from build123d import *

# Parameters (mm, degrees)
SKETCH2_W             = 152.4
SKETCH2_H             = 50.8
SKETCH2_W_2           = 146.05
SKETCH2_H_2           = 44.45
BOSS_EXTRUDE1_DEPTH   = 1133.475
BOSS_EXTRUDE1_2_DEPTH = 1133.475
BOSS_EXTRUDE4_DEPTH   = 858.8375
SKETCH5_W             = 50.8
SKETCH5_H             = 6.35
BOSS_EXTRUDE5_DEPTH   = 1163.6375
BOSS_EXTRUDE6_DEPTH   = 858.8375
SKETCH7_W             = 101.6
SKETCH7_H             = 101.6
BOSS_EXTRUDE7_DEPTH   = 25.4
SKETCH1_W             = 1143
SKETCH1_H             = 19.05
BOSS_EXTRUDE8_DEPTH   = 12.7
BOSS_EXTRUDE9_DEPTH   = 3.175
SKETCH8_R             = 6.35
CUT_EXTRUDE1_DEPTH    = 2252.98


with BuildPart() as part:
    # Sketch2 → Boss-Extrude1 (new body, symmetric)
    with BuildSketch(Plane(origin=(0, 0, 0), x_dir=(1, 0, 0), z_dir=(0, 1, 0))):
        with Locations((-505.61875, 0)):
            Rectangle(SKETCH2_W, SKETCH2_H)
        with Locations((-505.61875, 0)):
            Rectangle(SKETCH2_W_2, SKETCH2_H_2, mode=Mode.SUBTRACT)
    extrude(amount=BOSS_EXTRUDE1_DEPTH, both=True)



with BuildPart() as body_2:
    # Sketch2 → Boss-Extrude1 2 (new body, symmetric)
    with BuildSketch(Plane(origin=(0, 0, 0), x_dir=(1, 0, 0), z_dir=(0, 1, 0))):
        with Locations((505.61875, 0)):
            Rectangle(SKETCH2_W, SKETCH2_H)
        with Locations((505.61875, 0)):
            Rectangle(SKETCH2_W_2, SKETCH2_H_2, mode=Mode.SUBTRACT)
    extrude(amount=BOSS_EXTRUDE1_2_DEPTH, both=True)


with BuildPart() as part_1:
    add(part.part)

    add(body_2.part)  # Boss-Extrude4 merges body 2
    # Sketch3 → Boss-Extrude4 (add)
    with BuildSketch(Plane.ZY.offset(-429.41875)):
        Polygon((19.05, 987.425), (0, 987.425), (0, 981.075), (25.4, 981.075), (25.4, 1133.475), (-25.4, 1133.475), (-25.4, 1127.125), (19.05, 1127.125), align=None)
        Polygon((-25.4, -1133.475), (25.4, -1133.475), (25.4, -981.075), (0, -981.075), (0, -987.425), (19.05, -987.425), (19.05, -1127.125), (-25.4, -1127.125), align=None)
    extrude(amount=BOSS_EXTRUDE4_DEPTH)

    # Sketch5 → Boss-Extrude5 (add)
    with BuildSketch(Plane.ZY.offset(581.81875)):
        with Locations((0, -1133.475)):
            Rectangle(SKETCH5_W, SKETCH5_H)
        with Locations((0, 1133.475)):
            Rectangle(SKETCH5_W, SKETCH5_H)
    extrude(amount=-BOSS_EXTRUDE5_DEPTH)

    # Sketch6 → Boss-Extrude6 (add)
    with BuildSketch(Plane(origin=(-429.41875, 0, 0), x_dir=(0, 0, -1), z_dir=(1, 0, 0))):
        Polygon((-15.875, -981.075), (-15.875, -482.6), (6.35, -457.2), (6.35, -304.8), (-15.875, -279.4), (-15.875, 279.4), (6.35, 304.8), (6.35, 457.2), (-15.875, 482.6), (-15.875, 981.075), (-22.225, 981.075), (-22.225, 482.6), (0, 457.2), (0, 304.8), (-22.225, 279.4), (-22.225, -279.4), (0, -304.8), (0, -457.2), (-22.225, -482.6), (-22.225, -981.075), align=None)
    extrude(amount=BOSS_EXTRUDE6_DEPTH)

    # Sketch7 → Boss-Extrude7 (add)
    with BuildSketch(Plane.XY.offset(25.4)):
        with Locations((584.2, 1075.69)):
            Rectangle(SKETCH7_W, SKETCH7_H)
        with Locations((584.2, 364.49)):
            Rectangle(SKETCH7_W, SKETCH7_H)
        with Locations((584.2, -364.49)):
            Rectangle(SKETCH7_W, SKETCH7_H)
        with Locations((584.2, -1075.69)):
            Rectangle(SKETCH7_W, SKETCH7_H)
    extrude(amount=-BOSS_EXTRUDE7_DEPTH)

    # Sketch1 → Boss-Extrude8 (add)
    with BuildSketch(Plane.XY):
        with Locations((0, -1133.475)):
            Rectangle(SKETCH1_W, SKETCH1_H)
        with Locations((0, 1133.475)):
            Rectangle(SKETCH1_W, SKETCH1_H)
    extrude(amount=-BOSS_EXTRUDE8_DEPTH)

    # Sketch9 → Boss-Extrude9 (add)
    with BuildSketch(Plane.XY.offset(25.4)):
        with BuildLine():
            Line((635, 1126.49), (635, 1024.89))
            Line((635, 1024.89), (579.538518777, 1024.89))
            ThreePointArc((579.538518777, 1024.89), (572.213815984, 1026.468854084), (566.189972237, 1030.925013611))
            Line((566.189972237, 1030.925013611), (534.1840739, 1067.300724008))
            ThreePointArc((534.1840739, 1067.300724008), (531.01875, 1075.69), (534.1840739, 1084.079275992))
            Line((534.1840739, 1084.079275992), (566.189972237, 1120.454986389))
            ThreePointArc((566.189972237, 1120.454986389), (572.213815984, 1124.911145916), (579.538518777, 1126.49))
            Line((579.538518777, 1126.49), (635, 1126.49))
        make_face()
        with BuildLine():
            Line((635, 415.29), (635, 313.69))
            Line((635, 313.69), (578.904878784, 313.69))
            ThreePointArc((578.904878784, 313.69), (571.5, 315.30534194), (565.440611797, 319.857854871))
            Line((565.440611797, 319.857854871), (534.101416438, 356.195610622))
            ThreePointArc((534.101416438, 356.195610622), (531.01875, 364.49), (534.101416438, 372.784389378))
            Line((534.101416438, 372.784389378), (565.440611797, 409.122145129))
            ThreePointArc((565.440611797, 409.122145129), (571.5, 413.67465806), (578.904878784, 415.29))
            Line((578.904878784, 415.29), (635, 415.29))
        make_face()
        with BuildLine():
            Line((635, -313.69), (635, -415.29))
            Line((635, -415.29), (578.904878784, -415.29))
            ThreePointArc((578.904878784, -415.29), (571.5, -413.67465806), (565.440611797, -409.122145129))
            Line((565.440611797, -409.122145129), (534.101416438, -372.784389378))
            ThreePointArc((534.101416438, -372.784389378), (531.01875, -364.49), (534.101416438, -356.195610622))
            Line((534.101416438, -356.195610622), (565.440611797, -319.857854871))
            ThreePointArc((565.440611797, -319.857854871), (571.5, -315.30534194), (578.904878784, -313.69))
            Line((578.904878784, -313.69), (635, -313.69))
        make_face()
        with BuildLine():
            Line((635, -1024.89), (635, -1126.49))
            Line((635, -1126.49), (578.904878784, -1126.49))
            ThreePointArc((578.904878784, -1126.49), (571.5, -1124.87465806), (565.440611797, -1120.322145129))
            Line((565.440611797, -1120.322145129), (534.101416438, -1083.984389378))
            ThreePointArc((534.101416438, -1083.984389378), (531.01875, -1075.69), (534.101416438, -1067.395610622))
            Line((534.101416438, -1067.395610622), (565.440611797, -1031.057854871))
            ThreePointArc((565.440611797, -1031.057854871), (571.5, -1026.50534194), (578.904878784, -1024.89))
            Line((578.904878784, -1024.89), (635, -1024.89))
        make_face()
    extrude(amount=BOSS_EXTRUDE9_DEPTH)

    # Sketch8 → Cut-Extrude1 (cut)
    with BuildSketch(Plane(origin=(0, 1126.49, 0), x_dir=(1, 0, 0), z_dir=(0, 1, 0))):
        with Locations((619.91875, -12.7)):
            Circle(SKETCH8_R)
        with BuildLine():
            Line((619.91875, 0), (635, 0))
            Line((635, 0), (635, -28.575))
            Line((635, -28.575), (619.91875, -28.575))
            Line((619.91875, -28.575), (619.91875, -25.4))
            ThreePointArc((619.91875, -25.4), (632.61875, -12.7), (619.91875, 0))
        make_face()
    extrude(amount=-CUT_EXTRUDE1_DEPTH, mode=Mode.SUBTRACT)


solid = part_1.part
Work out the finished part from the listing and answer in its coordinate system (mm). A direction names the side the tool comes from. Give positions to 0.01 mm unless a question says otherwise; leave off trailing zeros. Write each loop counter-clockwise with the first axis right and the second up, starting at its lowest first coordinate (ties: lowest second). Pieces come first, ordered by that corner, then holes. Notation, with made-up numbers: M 48.5,27 L 96.5,27 A23 cw 96.5,56 Z; hole C -28.5,66.25 d10. An arc over 180 degrees is marked long. Answer as CSV lines item,"result".
Q1. A cutting plane is placed at A-A on y = -689.5. Write down the section's boundary in (x, z) (3 decimals).
A:
outline,"M -581.819,-25.4 L -429.419,-25.4 L -429.419,15.875 L 429.419,15.875 L 429.419,-25.4 L 581.819,-25.4 L 581.819,25.4 L 429.419,25.4 L 429.419,22.225 L -429.419,22.225 L -429.419,25.4 L -581.819,25.4 Z; hole M -578.644,-22.225 L -432.594,-22.225 L -432.594,22.225 L -578.644,22.225 Z; hole M 432.594,-22.225 L 578.644,-22.225 L 578.644,22.225 L 432.594,22.225 Z"
Q2. A tool of negligible diameter and unlimited length cuts with its end or side. For faces 5 (the flat face through (-6, -382, -6.35)), 6 (the flat face through (432.594, 16, 0)), 7 (the flat face through (586, 365, 28.575)), 8 (the flat face through (-6, -380, 0)), from which of +Z, -Z, +X, -X, +Y, -Y can it reach the whole face along a straight path? Write none if from no direction.
A:
face 5,"-Z"
face 6,"none"
face 7,"+Z, +X, -X, +Y, -Y"
face 8,"+Z"
Q3. The mould has two halves that part along Z. Classify faces 1 (the flat face through (581.819, 16, 0)), 2 (the flat face through (-6, -728, 22.225)), 3 (the flat face through (505, 1130.3, 5)), 4 (the flat face through (505, 16, 22.225)): +Z half, -Z half, draft (parallel to the pull), parting line (faces both ways), or undercut.
A:
face 1,"draft"
face 2,"+Z half"
face 3,"undercut"
face 4,"undercut"
Q4. Find the intervals of material crossed by probe 1 along X at (y, z) = (549.5, -1); probe 2 along X at (y, z) = (-521, 19); probe 3 along Y at (x, z) = (78, -11), in increasing order. Write a range as [from, to].
A:
probe 1,"x = [-581.82, -578.64], [-432.59, -429.42], [429.42, 432.59], [578.64, 581.82]"
probe 2,"x = [-581.82, -578.64], [-432.59, 432.59], [578.64, 581.82]"
probe 3,"y = [-1143, -1123.95], [1123.95, 1143]"
Q5. Given P1, Ø8, axis at x = -213, y = 519, coming from the -Z side (3 decimals); P2, Ø3, axis at y = 1140, z = -3.5, coming from the +X side; P3, Ø15, axis at x = 59.5, z = 10, coming from the -Y side, each flat-ended and moving along its own axis, determine where each tip first touches the part or whether it passes through.
A:
P1,"stops at z = 15.875"
P2,"stops at x = 571.5"
P3,"stops at y = -1136.65"
